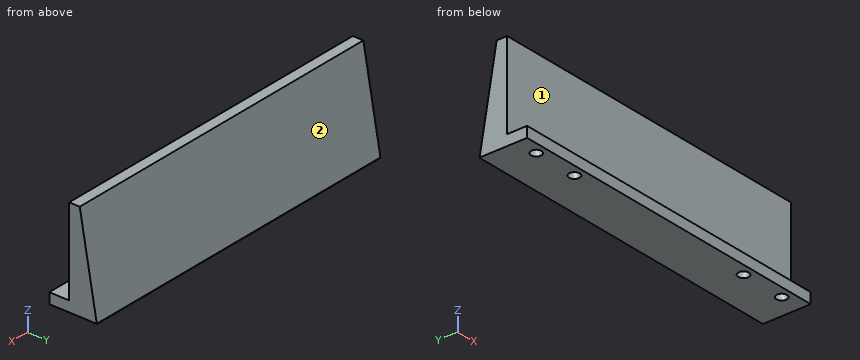
from build123d import *

# Parameters (mm, degrees)
SKETCH1_W           = 101.6
SKETCH1_H           = 26
BOSS_EXTRUDE1_DEPTH = 3.175
SKETCH2_W           = 101.6
SKETCH2_H           = 9.175
BOSS_EXTRUDE2_DEPTH = 3.175
SKETCH3_R           = 1.6
CUT_EXTRUDE1_DEPTH  = 3.175
BOSS_EXTRUDE3_DEPTH = 101.6


with BuildPart() as part:
    # Sketch1 → Boss-Extrude1 (new body)
    with BuildSketch(Plane(origin=(0, 0, 0), x_dir=(1, 0, 0), z_dir=(0, 1, 0))):
        Rectangle(SKETCH1_W, SKETCH1_H)
    extrude(amount=BOSS_EXTRUDE1_DEPTH)

    # Sketch2 → Boss-Extrude2 (add)
    with BuildSketch(Plane(origin=(0, 0, -13), x_dir=(-1, 0, 0), z_dir=(0, 0, -1))):
        with Locations((0, -1.4125)):
            Rectangle(SKETCH2_W, SKETCH2_H)
    extrude(amount=BOSS_EXTRUDE2_DEPTH)

    # Sketch3 → Cut-Extrude1 (cut)
    with BuildSketch(Plane.XY.offset(-13)):
        with Locations((30.3075, -3)):
            Circle(SKETCH3_R)
        with Locations((-30.3075, -3)):
            Circle(SKETCH3_R)
        with Locations((43.9685, -3)):
            Circle(SKETCH3_R)
        with Locations((-43.9685, -3)):
            Circle(SKETCH3_R)
    extrude(amount=-CUT_EXTRUDE1_DEPTH, mode=Mode.SUBTRACT)

    # Sketch4 → Boss-Extrude3 (add)
    with BuildSketch(Plane(origin=(50.8, 0, 0), x_dir=(0, 0, -1), z_dir=(1, 0, 0))):
        Polygon((16.175, 3.175), (16.175, 8.412812241), (16.143192443, 8.313731132), (-13, 3.175), align=None)
    extrude(amount=-BOSS_EXTRUDE3_DEPTH)


solid = part.part
Here's how the part is built. I have some questions about the finished solid (model axes, mm). Face numbers are marked on the shaded views. A direction names the side the tool comes from. Coordinates: 2 decimals unless noted, no trailing zeros. Loops run counter-clockwise (first coordinate to the right, second up) from the corner with the lowest first, then second, coordinate; pieces in that order, holes last. Notation, with made-up numbers: (73.25, 37.25) -> (88.25, 37.25) arc R15 cw to (88.25, 64.25) -> close; hole circle Ø1 at (21.5, 57.25). An arc over 180 degrees is marked (long way). Use one line per item in the form item = value. Start each with the question number.
(1) If we section it at A-A (y = -3): Please give me the cut outline in (x, z) (1 decimal).
(2) If we section it at B-B (x = -6): Please give me the cut outline in (y, z) (3 decimals), then the cut area to 3 significant figures.
(3) On a 3-axis mill with a long thin cutter (end or side, diameter ignored), from which of +Z, -Z, +X, -X, +Y, -Y can I reach the whole of each face in a straight line? I mean the marked faces 1 and 2. Say none if no direction works.
(4) If we section it at D-D (z = 5.5): Please give me the cut outline in (x, y).
(5) Will these pins go through, and if not, where does the flat tip stop? pin 1 (4 mm diameter, centred on x = 43.97, y = -3, fed in from +Z); pin 2 (1 mm diameter, centred on x = -13.5, z = 2, fed in from -Y); pin 3 (1 mm diameter, centred on x = -37.5, z = -10.5, fed in from +Y).
(6) If we section it at C-C (y = 7.25): Please give me the cut outline in (x, z) (3 decimals).
(7) Please list where these lines run through material, in increasing order: line 1 along Z through (x, y) = (33.5, -1.5) (3 decimals); line 2 along Y through (x, z) = (29.5, 3.25); line 3 along Y through (x, z) = (14.5, -11).
Verdict:
q1.outline = (-50.8, -16.2) -> (-45.6, -16.2) -> (-45.6, -13) -> (-50.8, -13) -> close; (-42.4, -16.2) -> (-31.9, -16.2) -> (-31.9, -13) -> (-42.4, -13) -> close; (-28.7, -16.2) -> (28.7, -16.2) -> (28.7, -13) -> (-28.7, -13) -> close; (31.9, -16.2) -> (42.4, -16.2) -> (42.4, -13) -> (31.9, -13) -> close; (45.6, -16.2) -> (50.8, -16.2) -> (50.8, -13) -> (45.6, -13) -> close
q2.outline = (-6, -16.175) -> (8.413, -16.175) -> (8.314, -16.143) -> (3.175, 13) -> (0, 13) -> (0, -13) -> (-6, -13) -> close
q2.area = 187 mm²
q3.face_1 = +Z, +X, -X, -Y
q3.face_2 = +Z, +X, -X, +Y
q4.outline = (-50.8, 0) -> (50.8, 0) -> (50.8, 4.5) -> (-50.8, 4.5) -> close
q5.pin_1 = -13
q5.pin_2 = 0
q5.pin_3 = 7.41
q6.outline = (-50.8, -16.175) -> (50.8, -16.175) -> (50.8, -10.11) -> (-50.8, -10.11) -> close
q7.line_1 = -16.175 to -13
q7.line_2 = 0 to 4.89
q7.line_3 = 0 to 7.41
